Source: CAD feature listing. Evaluate the final solid. Frame: model axes, mm. Face numbers are marked on the shaded views. A direction names the side the tool comes from. Coordinates: 2 decimals unless noted, no trailing zeros. Loops run counter-clockwise (first coordinate to the right, second up) from the corner with the lowest first, then second, coordinate; pieces in that order, holes last. Notation, with made-up numbers: (82.5, 76.25) - (94.5, 76.25) arc R29 ccw to (94.5, 114.25) - close; hole circle Ø8 at (-34.5, 29). An arc over 180 degrees is marked (long way). Write item = value, one per line. Start each with the question number.
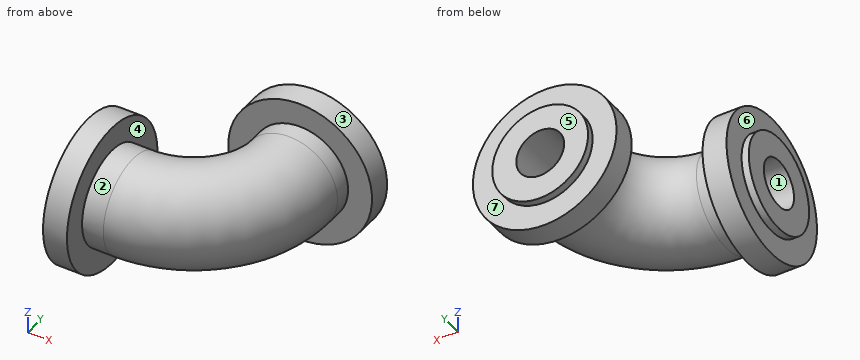
from build123d import *

# Parameters (mm, degrees)
F0_R     = 20
F0_R_2   = 10
F4_R     = 30
F4_R_2   = 20
F5_DEPTH = 10
F7_R     = 30
F7_R_2   = 20
F8_DEPTH = 10


with BuildPart() as f2:
    # F2: sweep along a path in F1
    with BuildLine(Plane.XY) as f2_path:
        Line((0, 0), (0, -20))
        ThreePointArc((0, -20), (-11.7157287525, -48.2842712475), (-40, -60))
        Line((-40, -60), (-61.8760055131, -60))
    # F0 (on Front) → F2 (sweep)
    with BuildSketch(Plane.XZ):
        Circle(F0_R)
        Circle(F0_R_2, mode=Mode.SUBTRACT)
    sweep(path=f2_path.line)

    # F4 (on offset) → F5 (join)
    with BuildSketch(Plane(origin=(-58.8760055131, 0, 0), x_dir=(0, -1, 0), z_dir=(-1, 0, 0))):
        with Locations((60, 0)):
            Circle(F4_R)
        with Locations((60, 0)):
            Circle(F4_R_2, mode=Mode.SUBTRACT)
    extrude(amount=-F5_DEPTH)

    # F7 (on offset) → F8 (join)
    with BuildSketch(Plane(origin=(0, -3, 0), x_dir=(-1, 0, 0), z_dir=(0, 1, 0))):
        Circle(F7_R)
        Circle(F7_R_2, mode=Mode.SUBTRACT)
    extrude(amount=-F8_DEPTH)


solid = f2.part
Item 1: Cut plane B-B (x = -50.5). Return the cut outline in (y, z).
Item 2: Reachability of the marked faces 4, 5, 6 and 7 from +Z, -Z, +X, -X, +Y, -Y: full face, straight path, thin tool, end or side. Return the list, or none.
Item 3: Cut plane C-C (z = 12). Return the cut outline in (x, y), then the cut area to 3 significant figures.
Item 4: Material intervals for L1, parallel to Z at x = -53, y = -60; L2, parallel to Z at x = 0, y = -13.25; L3, parallel to Y at x = -29.5, z = 5, sorted ascending. Write a range as [from, to].
Item 5: Draft query along Y for the marked faces 1, 2 and 3. Return one class per face: released by +Y, released by -Y, zero draft, split by the parting line, or undercut.
Item 6: First-contact query: pin 1 (2 mm diameter, centred on y = -73, z = -18, fed in from -X); pin 2 (1 mm diameter, centred on x = -52, z = -23, fed in from +Y); pin 3 (12 mm diameter, centred on x = 0, z = 0, fed in from +Y). Flat tips, straight axial feed; report the tip coordinate or a pass-through.
Responses:
q1.outline = circle Ø60 at (-60, 0); hole circle Ø20 at (-60, 0)
q2.face_4 = none
q2.face_5 = +Z, -Z, +X, -X, +Y
q2.face_6 = -X
q2.face_7 = +Y
q3.outline = (-61.88, -76) - (-58.88, -76) - (-58.88, -87.5) - (-48.88, -87.5) - (-48.88, -76) - (-40, -76) arc R56 ccw to (16, -20) - (16, -13) - (27.5, -13) - (27.5, -3) - (16, -3) - (16, 0) - (-16, 0) - (-16, -3) - (-27.5, -3) - (-27.5, -13) - (-16, -13) - (-16, -20) arc R24 cw to (-40, -44) - (-48.88, -44) - (-48.88, -32.5) - (-58.88, -32.5) - (-58.88, -44) - (-61.88, -44) - close
q3.area = 3,810 mm2
q4.L1 = [-30, -10], [10, 30]
q4.L2 = [-20, -10], [10, 20]
q4.L3 = [-78.43, -67.51], [-49.53, -37.76], [-13, -3]
q5.face_1 = undercut
q5.face_2 = split by the parting line
q5.face_3 = zero draft
q6.pin_1 = -58.88
q6.pin_2 = -40.16
q6.pin_3 = -39.6
